from build123d import *


with BuildPart() as part:
    # Sketch1 → Revolve1 (revolve)
    with BuildSketch(Plane.XY, mode=Mode.PRIVATE) as revolve1_sk:
        with BuildLine():
            Line((1, -2), (1, 2.5))
            Line((1, 2.5), (12, 2.5))
            Line((12, 2.5), (12, 3.5))
            Line((12, 3.5), (15, 3.5))
            Line((15, 3.5), (15, 2.5))
            ThreePointArc((15, 2.5), (16.25, 1.25), (15, 0))
            Line((15, 0), (15, -1))
            Line((15, -1), (12, -1))
            Line((12, -1), (12, 0))
            Line((12, 0), (3, 0))
            Line((3, 0), (3, -2))
            Line((3, -2), (1, -2))
        make_face()
    revolve(revolve1_sk.sketch.rotate(Axis((0, 26.353801269, 0), (0, -1, 0)), 90), axis=Axis((0, 26.353801269, 0), (0, -1, 0)))


solid = part.part
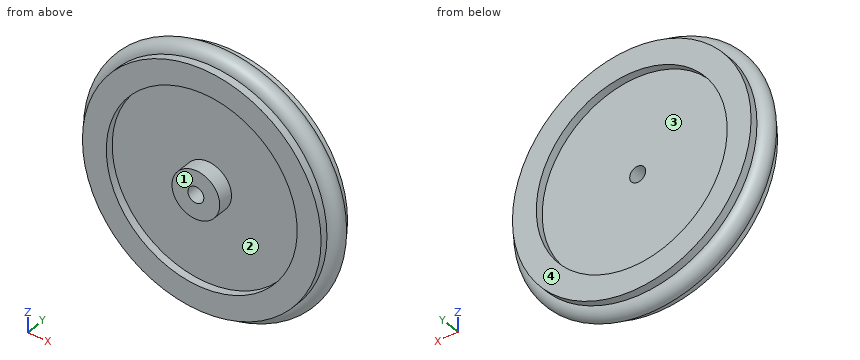
CAD build for the part. Positions are in the model's coordinates, mm. Face numbers are marked on the shaded views. A direction names the side the tool comes from. Round coordinates to 2 decimals unless told otherwise and drop trailing zeros. Write each loop counter-clockwise with the first axis right and the second up, starting at its lowest first coordinate (ties: lowest second). Pieces come first, ordered by that corner, then holes. Notation, with made-up numbers: (37, 71) -> (92, 71) arc R25 cw to (92, 103) -> close; hole circle Ø10 at (76.5, 1.25). An arc over 180 degrees is marked (long way). Answer as a JSON object with one key per item and string values.
(1) Two-plate mould, pull along Z, no slides. Class the marked faces 1 and 2: +Z half, -Z half, draft (parallel to the pull), parting line (faces both ways), or undercut.
Reported:
{"face 1": "draft", "face 2": "undercut"}
(2) Which spindle directions (+Z, -Z, +X, -X, +Y, -Y) get a long thin tool onto all of the face, cutting with end or side? Do the marked faces 3 and 4. Say none if no direction does.
Reported:
{"face 3": "+Y", "face 4": "+Z, -Z, +X, -X, +Y"}
(3) Band-saw the part on C-C, the plane y = 2. List the corners of the cut face in (x, z).
Reported:
{"outline": "circle Ø32 at (0, 0); hole circle Ø2 at (0, 0)"}
(4) Pin check, flat tips, straight feed: P1, Ø5, axis at x = -1, z = -3, coming from the +Y side; P2, Ø12, axis at x = 9, z = 4, coming from the -Y side; P3, Ø1, axis at x = -10.5, z = 0.5, coming from the -Y side; P4, Ø15, axis at x = -5, z = -1, coming from the -Y side. Stop position of each tip, or through.
Reported:
{"P1": "stops at y = 2.5", "P2": "stops at y = -1", "P3": "stops at y = 0", "P4": "stops at y = -2"}
(5) Probe probe 1 along X at (y, z) = (3.15, 0); probe 2 along Z at (x, y) = (-7, 3.05); probe 3 along Y at (x, z) = (9.5, 3). List the from-to ranges inside material, lowest first. Write a range as [from, to].
Reported:
{"probe 1": "x = [-15, -12], [12, 15]", "probe 2": "z = [-13.27, -9.75], [9.75, 13.27]", "probe 3": "y = [0, 2.5]"}
(6) Band-saw the part on A-A, the plane x = 0. List the corners of the cut face in (y, z).
Reported:
{"outline": "(-2, -3) -> (0, -3) -> (0, -12) -> (-1, -12) -> (-1, -15) -> (0, -15) arc R1.25 ccw to (2.5, -15) -> (3.5, -15) -> (3.5, -12) -> (2.5, -12) -> (2.5, -1) -> (-2, -1) -> close; (-2, 1) -> (2.5, 1) -> (2.5, 12) -> (3.5, 12) -> (3.5, 15) -> (2.5, 15) arc R1.25 ccw to (0, 15) -> (-1, 15) -> (-1, 12) -> (0, 12) -> (0, 3) -> (-2, 3) -> close"}
(7) Band-saw the part on B-B, the plane z = 0. List the corners of the cut face in (x, y), then the cut area to 3 significant figures.
Reported:
{"outline": "(-15, -1) -> (-12, -1) -> (-12, 0) -> (-3, 0) -> (-3, -2) -> (-1, -2) -> (-1, 2.5) -> (-12, 2.5) -> (-12, 3.5) -> (-15, 3.5) -> (-15, 2.5) arc R1.25 ccw to (-15, 0) -> close; (1, -2) -> (3, -2) -> (3, 0) -> (12, 0) -> (12, -1) -> (15, -1) -> (15, 0) arc R1.25 ccw to (15, 2.5) -> (15, 3.5) -> (12, 3.5) -> (12, 2.5) -> (1, 2.5) -> close", "area": "94.9 mm^2"}
